Autodesk Inventor part; units mm, degrees
ref_plane "YZ Plane" through (0, 0, 0) normal (1, 0, 0) x (0, 1, 0)
ref_plane "XZ Plane" through (0, 0, 0) normal (0, 1, 0) x (-1, 0, 0)
ref_plane "XY Plane" through (0, 0, 0) normal (0, 0, 1) x (1, 0, 0)
sketch "Sketch4" plane through (0, 0, 0) normal (0, 1, 0) x (-1, 0, 0)
  line L0 (0, 0) -> (-42, 0)
  line L1 (-42, 0) -> (-42, -52)
  line L2 (-42, -52) -> (0, -52)
  line L3 (0, -52) -> (0, 0)
  dimension "d79" = 42
  dimension "d80" = 52
extrude "Extrusion4" add sketch "Sketch4" along normal blind 15
sketch "Sketch5" plane through (0, 15, 0) normal (0, 1, 0) x (1, 0, 0)
  line L0 (0, 0) -> (0, 10)
  line L1 (0, 52) -> (0, 0)
  line L2 (0, 52) -> (0, 42)
  circle A0 centre (16, 26) radius 16
  line L3 (42, 0) -> (42, 52)
  line L4 (0, 10) -> (42, 10)
  line L5 (0, 42) -> (42, 42)
  point P0 (42, 26)
  point P1 (16, 10)
  point P2 (16, 42)
  dimension "d83" = 10
  dimension "d84" = 10
  dimension "d93" = 32
  dimension "d94" = 26
extrude "Extrusion5" cut sketch "Sketch5" against normal blind 15 contours L5 A0 L1 | A0 L4 L1 | A0
sketch "Sketch10" plane through (42, 0, 0) normal (1, 0, 0) x (0, 0, -1)
  circle A0 centre (5, 7.5) radius 2.65
  line L0 (18.9423, 0.7517) -> (33.0845, 14.8938)
  line L1 (0, 0) -> (52, 0)
  line L2 (26, 0) -> (26, 15)
  line L3 (0, 15) -> (52, 15)
  line L4 (18.9423, 0.7517) -> (26.0134, 7.8228)
  circle A1 centre (18.9423, 0.7517) radius 1.55
  circle A2 centre (33.0845, 14.8938) radius 1.55
  circle A3 centre (33.0845, 14.8938) radius 5
  circle A4 centre (18.9423, 0.7517) radius 5
  line L5 (52, 0) -> (0, 0)
  point P0 (38.0833, 15)
  point P1 (28.0856, 15)
  point P2 (31.5381, 15)
  point P3 (34.6308, 15)
  point P4 (13.9992, 0)
  point P5 (23.8855, 0)
  point P6 (20.2979, 0)
  point P7 (17.5868, 0)
  point P8 (47, 7.5)
  dimension "d115" = 20
  dimension "d116" = 3.1
  dimension "d117" = 3.1
  dimension "d118" = 10
  dimension "d119" = 10
extrude "Extrusion10" add sketch "Sketch10" against normal blind 10 contours A1 L1 A4 | A3 L3 A2
sketch "Sketch11" plane through (42, 0, 0) normal (1, 0, 0) x (0, 0, -1)
  arc A0 (34.6308, 15) -> (31.5381, 15) centre (33.0845, 14.8938) ccw
  circle A1 centre (33.0845, 14.8938) radius 1.55
  point P0 (0, 0)
  point P1 (31.5381, 15)
  point P2 (34.6308, 15)
  dimension "d122" = 3.1
extrude "Extrusion11" cut sketch "Sketch11" against normal blind 30
sketch "Sketch12" plane through (42, 0, 0) normal (1, 0, 0) x (0, 0, -1)
  circle A0 centre (33.0845, 14.8938) radius 1.55
  circle A1 centre (33.0845, 14.8938) radius 3
  point P0 (0, 0)
  dimension "d125" = 6
extrude "Extrusion12" cut sketch "Sketch12" against normal blind 30
sketch "Sketch13" plane through (42, 0, 0) normal (1, 0, 0) x (0, 0, -1)
  circle A0 centre (33.0845, 14.8938) radius 3
  circle A1 centre (33.0845, 14.8938) radius 1.625
  point P0 (0, 0)
  dimension "d128" = 3.25
extrude "Extrusion13" add sketch "Sketch13" against normal blind 5
sketch "Sketch14" plane through (42, 0, 0) normal (1, 0, 0) x (0, 0, -1)
  arc A0 (17.5868, 0) -> (20.2979, 0) centre (18.9423, 0.7517) ccw
  circle A1 centre (18.9423, 0.7517) radius 3
  point P0 (0, 0)
  dimension "d131" = 6
extrude "Extrusion14" cut sketch "Sketch14" against normal blind 16
sketch "Sketch15" plane through (42, 0, 0) normal (1, 0, 0) x (0, 0, -1)
  circle A0 centre (18.9423, 0.7517) radius 1.625
  circle A1 centre (18.9423, 0.7517) radius 2.65
  point P0 (0, 0)
  dimension "d134" = 3.25
extrude "Extrusion15" add sketch "Sketch15" against normal blind 5
sketch "Sketch16" plane through (42, 0, -52) normal (1, 0, 0) x (0, 0, -1)
  arc A0 (-20.2979, 0) -> (-17.5868, 0) centre (-18.9423, 0.7517) ccw
  circle A1 centre (-18.9423, 0.7517) radius 1.55
  point P0 (-52, 0)
sketch "Sketch18" plane through (0, 0, 0) normal (0, -1, 0) x (1, 0, 0)
  line L0 (0, -10) -> (0, 0)
  line L1 (0, -5) -> (9, -5)
  circle A0 centre (9, -5) radius 1.625
  line L2 (0, -52) -> (0, -42)
  line L3 (0, -47) -> (9, -47)
  circle A1 centre (9, -47) radius 1.625
  dimension "d144" = 9
  dimension "d145" = 3.25
  dimension "d146" = 9
  dimension "d147" = 3.25
extrude "Extrusion17" cut sketch "Sketch18" against normal blind 26.5
sketch "Sketch19" plane through (42, 0, 0) normal (1, 0, 0) x (0, 0, -1)
  point P0 (0, 0)
sketch "Sketch20" plane through (42, 0, 0) normal (1, 0, 0) x (0, 0, -1)
  point P0 (0, 0)
sketch "Sketch21" plane through (42, 0, 0) normal (1, 0, 0) x (0, 0, -1)
  line L0 (52, 0) -> (42, 0)
  line L1 (10, 15) -> (0, 15)
  line L2 (52, 0) -> (0, 0)
  line L3 (0, 0) -> (0, 15)
  line L4 (0, 15) -> (52, 15)
  line L5 (52, 15) -> (52, 0)
  circle A0 centre (18.9423, 0.7517) radius 1.625
  circle A1 centre (18.9423, 0.7517) radius 1.625
  circle A2 centre (33.0845, 14.8938) radius 1.625
  circle A3 centre (33.0845, 14.8938) radius 1.625
  arc A4 (38.0833, 15) -> (28.0856, 15) centre (33.0845, 14.8938) ccw
  circle A5 centre (33.0845, 14.8938) radius 5
  arc A6 (13.9992, 0) -> (23.8855, 0) centre (18.9423, 0.7517) ccw
  circle A7 centre (18.9423, 0.7517) radius 5
  dimension "d150" = 3.25
extrude "Extrusion18" add sketch "Sketch21" along normal blind 33 contours L0 L2 A7 L3 L1 L4 A5 L5 | A6 L2 A0 | L2 A0 A7 | A5 L4 A2 | L4 A2 A4
sketch "Sketch22" plane through (37, 0.7517, -18.9423) normal (-1, 0, 0) x (0, 0, 1)
  circle A0 centre (0, 0) radius 3
  circle A1 centre (0, 0) radius 3
  point P0 (18.9423, -0.7517)
  dimension "d153" = 6
extrude "Extrusion19" cut sketch "Sketch22" against normal blind 33
sketch "Sketch23" plane through (37, 14.8938, -33.0845) normal (-1, 0, 0) x (0, 0, 1)
  arc A0 (4.9989, 0.1062) -> (-4.9989, 0.1062) centre (0, 0) ccw
  circle A1 centre (0, 0) radius 3
  point P0 (33.0845, -14.8938)
  dimension "d156" = 6
extrude "Extrusion20" cut sketch "Sketch23" against normal blind 33
properties part number "braket motor1"
Verification items for the finished model (mm, model axes). A direction names the side the tool comes from. Coordinates: 2 decimals unless noted, no trailing zeros. Write each loop counter-clockwise with the first axis right and the second up, starting at its lowest first coordinate (ties: lowest second). Pieces come first, ordered by that corner, then holes. Notation, with made-up numbers: (71.5, 30) -> (97.5, 30) arc R24 ccw to (97.5, 50) -> close; hole circle Ø10 at (-35, 13.25). An arc over 180 degrees is marked (long way). One line per item, written item: value. Start each with the question number.
Q1. Access from +Z, -Z, +X, -X, +Y, -Y to the whole of each face (thin tool, end or side, straight path). Record for faces 1 (the flat face through (70, 13.6, -31.8)), 2 (the flat face through (32, -3, -19)), 3 (the cylindrical face through (72.46, 14.82, -31.46)), 4 (the flat face through (8, 8, -42)).
Q2. Cross-section at C-C on x = 39.5. Enter the section's corners in (y, z), and give its area (3 significant figures).
Q3. Cross-section at D-D on z = -37. Enter the section's corners in (x, y).
Q4. Go/stop test with flat-tipped pins: P1, Ø2.5, axis at x = 9, z = -47, coming from the +Y side; P2, Ø1.3, axis at y = -1.5, z = -17, coming from the -X side; P3, Ø17.5, axis at x = 17, z = -47.5, coming from the +Y side; P4, Ø5, axis at x = 14, z = -7, coming from the -Y side. Record where each tip stops, or that it passes through.
Q5. Thickness scan on L1, parallel to Z at x = 9, y = 3.5 (3 decimals); L2, parallel to Z at x = 4, y = 8; L3, parallel to Y at x = 40, z = -2. Record the ranges inside material, lowest first. Write a range as from..to.
Q6. Cross-section at A-A on z = -5. Enter the section's corners in (x, y) (3 decimals), and give its area (3 significant figures).
Q7. Mould release check, pull along Y, two halves, no side actions. Record for faces 5 (the flat face through (32, 19, -33)), 6 (the cylindrical face through (37.07, 19.893, -33.193)), 7 (the flat face through (70, -1, -18)): pulls with the +Y half, pulls with the -Y half, needs draft (parallel to the pull), parting line crosses it, or undercut.
Q8. Cross-section at B-B on x = 9. Enter the section's corners in (y, z) (3 decimals).
Checked values:
1. face 1: -X
1. face 2: +Z, -Z, -X, -Y
1. face 3: +X, -X
1. face 4: -X, +Y, -Y
2. outline: (0, -52) -> (15, -52) -> (15, -38.08) arc R5 ccw to (15, -28.09) -> (15, 0) -> (0, 0) -> (0, -14) arc R5 ccw to (0, -23.89) -> close; hole circle Ø6 at (0.75, -18.94); hole circle Ø6 at (14.89, -33.08)
2. area: 793 mm²
3. outline: (27.62, 0) -> (75, 0) -> (75, 18) -> (32, 18) -> (32, 15) -> (27.62, 15) -> close
4. P1: passes through
4. P2: stops at x = 32
4. P3: stops at y = 15
4. P4: stops at y = 0
5. L1: z = -52..-48.625, -45.375..-42, -10..-6.625, -3.375..0
5. L2: z = -52..-42, -10..0
5. L3: y = 0..15
6. outline: (0, 0) -> (7.375, 0) -> (7.375, 15) -> (0, 15) -> close; (10.625, 0) -> (75, 0) -> (75, 15) -> (10.625, 15) -> close
6. area: 1,080 mm²
7. face 5: needs draft
7. face 6: pulls with the +Y half
7. face 7: undercut
8. outline: (0, -52) -> (15, -52) -> (15, -48.625) -> (0, -48.625) -> close; (0, -45.375) -> (15, -45.375) -> (15, -42) -> (0, -42) -> close; (0, -10) -> (15, -10) -> (15, -6.625) -> (0, -6.625) -> close; (0, -3.375) -> (15, -3.375) -> (15, 0) -> (0, 0) -> close
